Read the model definition and answer for the solid it produces. Units are mm, in the model's axes. Face numbers are marked on the shaded views. A direction names the side the tool comes from. Round coordinates to 2 decimals unless told otherwise and drop trailing zeros. Write each loop counter-clockwise with the first axis right and the second up, starting at its lowest first coordinate (ties: lowest second). Pieces come first, ordered by that corner, then holes. Notation, with made-up numbers: (32, 75.5) -> (74, 75.5) arc R25 cw to (74, 109.5) -> close; hole circle Ø8 at (41, 63). An arc over 180 degrees is marked (long way). Return JSON: item names as keys, results as strings. Group by question number.
(1) Given pin 1 (5.5 mm diameter, centred on y = 7, z = 32, fed in from +X); pin 2 (5.5 mm diameter, centred on x = 7.5, z = 29, fed in from +Y); pin 3 (20 mm diameter, centred on x = 33, y = 10.5, fed in from -Z), each flat-ended and moving along its own axis, determine where each tip first touches the part or whether it passes through.
(2) For the marked faces 1, 2 and 3, determine the directions among +Z, -Z, +X, -X, +Y, -Y from which every point of the face is accessible in a straight line to the end or side of a thin tool.
(3) A cutting plane is placed at C-C on y = 26. Give the vertices of the cut face in (x, z).
(4) A straight line is drawn through the part: line 1 (Y direction, x = 26, z = 10.5). Find the intervals that lie inside material, in ascending order.
(5) A cutting plane is placed at A-A on z = 3.5. Give the vertices of the cut face in (x, y), then the cut area to 3 significant figures.
```python
from build123d import *

# Parameters (mm, degrees)
BOX003_W     = 18
BOX003_H     = 18
BOX003_DEPTH = 18
BOX002_W     = 18
BOX002_H     = 18
BOX002_DEPTH = 18
BOX001_W     = 18
BOX001_H     = 18
BOX001_DEPTH = 18
BOX_W        = 20
BOX_H        = 20
BOX_DEPTH    = 20


with BuildPart() as z:
    # Box003 → Box003 (new body)
    with BuildSketch(Plane(origin=(1, 1, 20), x_dir=(1, 0, 0), z_dir=(0, 0, 1))):
        with Locations((9, 9)):
            Rectangle(BOX003_W, BOX003_H)
    extrude(amount=BOX003_DEPTH)


with BuildPart() as y:
    # Box002 → Box002 (new body)
    with BuildSketch(Plane(origin=(1, 20, 1), x_dir=(1, 0, 0), z_dir=(0, 0, 1))):
        with Locations((9, 9)):
            Rectangle(BOX002_W, BOX002_H)
    extrude(amount=BOX002_DEPTH)


with BuildPart() as x:
    # Box001 → Box001 (new body)
    with BuildSketch(Plane(origin=(20, 1, 1), x_dir=(1, 0, 0), z_dir=(0, 0, 1))):
        with Locations((9, 9)):
            Rectangle(BOX001_W, BOX001_H)
    extrude(amount=BOX001_DEPTH)


with BuildPart() as unionxyz:
    # Box → Box (new body)
    with BuildSketch(Plane.XY):
        with Locations((10, 10)):
            Rectangle(BOX_W, BOX_H)
    extrude(amount=BOX_DEPTH)

    # Fusion: union X
    add(x.part)

    # Fusion001: union Y
    add(y.part)

    # Fusion002: union Z
    add(z.part)


solid = unionxyz.part
```
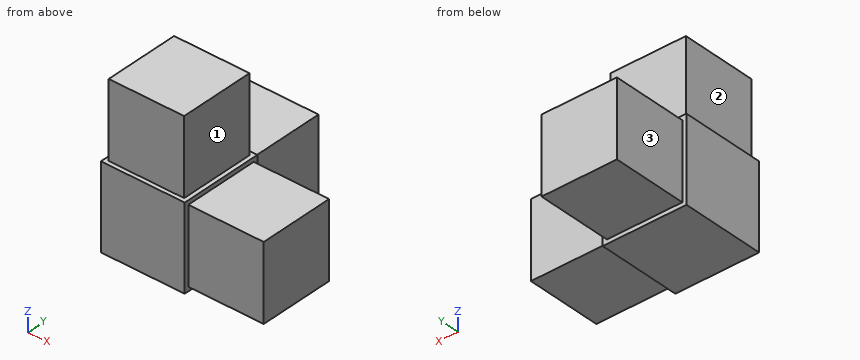
Checks:
{
 "1": {"pin 1": "stops at x = 19", "pin 2": "stops at y = 19", "pin 3": "stops at z = 1"},
 "2": {"face 1": "+Z, +X, +Y, -Y", "face 2": "+Z, -X, +Y, -Y", "face 3": "+Z, -Z, -X, +Y"},
 "3": {"outline": "(1, 1) -> (19, 1) -> (19, 19) -> (1, 19) -> close"},
 "4": {"line 1": "y = 1 to 19"},
 "5": {"outline": "(0, 0) -> (20, 0) -> (20, 1) -> (38, 1) -> (38, 19) -> (20, 19) -> (20, 20) -> (19, 20) -> (19, 38) -> (1, 38) -> (1, 20) -> (0, 20) -> close", "area": "1,050 mm^2"}
}
